Part model, mm, in its own coordinate system. A direction names the side the tool comes from. Coordinates: 2 decimals unless noted, no trailing zeros. Write each loop counter-clockwise with the first axis right and the second up, starting at its lowest first coordinate (ties: lowest second). Pieces come first, ordered by that corner, then holes. Notation, with made-up numbers: (2.5, 43.25) - (30.5, 43.25) arc R10 cw to (30.5, 50.25) - close; hole circle Ø2 at (-2, 5.25). An arc over 180 degrees is marked (long way). Write each question's results on one line, items separated by ' | '.
from build123d import *

# Parameters (mm, degrees)
SKETCH_W     = 108
SKETCH_H     = 75.2
PAD_DEPTH    = 2
SKETCH001_R  = 1.55
POCKET_DEPTH = 2
SKETCH002_W  = 10
SKETCH002_H  = 10
PAD001_DEPTH = 60
PAD002_DEPTH = 10
PAD003_DEPTH = 10
PAD004_DEPTH = 10
SKETCH003_W  = 10
SKETCH003_H  = 10
PAD005_DEPTH = 60
PAD006_DEPTH = 10
FILLET_R     = 1
FILLET001_R  = 1
FILLET002_R  = 1
FILLET003_R  = 1
BOX_W        = 108
BOX_H        = 75.2
BOX_DEPTH    = 10
BOX001_W     = 216
BOX001_H     = 150.4
BOX001_DEPTH = 30


with BuildPart() as part:
    # Sketch → Pad (new body)
    with BuildSketch(Plane.XY):
        Rectangle(SKETCH_W, SKETCH_H)
    extrude(amount=PAD_DEPTH)

    # Sketch001 (on Face6 of Pad) → Pocket (cut)
    with BuildSketch(Plane.XY.offset(2)):
        with Locations((-49.75, 33.05)):
            Circle(SKETCH001_R)
        with Locations((49.75, 33.05)):
            Circle(SKETCH001_R)
        with Locations((49.75, -33.05)):
            Circle(SKETCH001_R)
        with Locations((-49.75, -33.05)):
            Circle(SKETCH001_R)
    extrude(amount=-POCKET_DEPTH, mode=Mode.SUBTRACT)

    # Sketch002 (on Face5 of Pocket) → Pad001 (join)
    with BuildSketch(Plane(origin=(-14.437445, 5.037445, 35.081278), x_dir=(0.866025, 0, 0.5), z_dir=(-0.433013, 0.5, 0.75))):
        with Locations((-32.6, 32.6)):
            Rectangle(SKETCH002_W, SKETCH002_H)
    pad001 = extrude(amount=PAD001_DEPTH)

    # Mirrored: Pad001 across YZ
    add(pad001.mirror(Plane.YZ))

    # Mirrored001: Pad001 across XZ
    add(pad001.mirror(Plane.XZ))

    # Mirrored001 Face22 → Pad002 (add)
    with BuildSketch(Plane(origin=(34.284733, 32.964866, 5.00416), x_dir=(-0.755929, 0.654654, 0), z_dir=(-0.433013, -0.5, -0.75))):
        Polygon((3.146916, 4.541863), (-2.963185, 4.541863), (-7.030988, 1.019042), (-0.484451, -6.540247), (7.074838, 0.006289), align=None)
    extrude(amount=PAD002_DEPTH)

    # Pad002 Face21 → Pad003 (add)
    with BuildSketch(Plane(origin=(-34.284733, 32.964866, 5.00416), x_dir=(-0.755929, -0.654654, 0), z_dir=(0.433013, -0.5, -0.75))):
        Polygon((2.963185, 4.541863), (-3.146916, 4.541863), (-7.074838, 0.006289), (0.484451, -6.540247), (7.030988, 1.019042), align=None)
    extrude(amount=PAD003_DEPTH)

    # Pad003 Face35 → Pad004 (add)
    with BuildSketch(Plane(origin=(-34.284733, -32.964866, 5.00416), x_dir=(0.755929, -0.654654, 0), z_dir=(0.433013, 0.5, -0.75))):
        Polygon((3.146916, 4.541863), (-2.963185, 4.541863), (-7.030988, 1.019042), (-0.484451, -6.540247), (7.074838, 0.006289), align=None)
    extrude(amount=PAD004_DEPTH)

    # Sketch003 (on Face4 of Pad004) → Pad005 (join)
    with BuildSketch(Plane(origin=(14.437445, -5.037445, 35.081278), x_dir=(0.866025, 0, -0.5), z_dir=(0.433013, -0.5, 0.75))):
        with Locations((32.6, -32.6)):
            Rectangle(SKETCH003_W, SKETCH003_H)
    extrude(amount=PAD005_DEPTH)

    # Pad005 Face44 → Pad006 (add)
    with BuildSketch(Plane(origin=(34.284733, -32.964866, 5.00416), x_dir=(0.755929, 0.654654, 0), z_dir=(-0.433013, 0.5, -0.75))):
        Polygon((-7.074838, 0.006289), (0.484451, -6.540247), (7.030988, 1.019042), (2.963185, 4.541863), (-3.146916, 4.541863), align=None)
    extrude(amount=PAD006_DEPTH)

    # Fillet
    fillet_edges = [part.edges().sort_by_distance(p)[0] for p in [
        (-54, -37.6, 1),
    ]]
    fillet(fillet_edges, radius=FILLET_R)

    # Fillet001
    fillet001_edges = [part.edges().sort_by_distance(p)[0] for p in [
        (-54, 37.6, 1),
    ]]
    fillet(fillet001_edges, radius=FILLET001_R)

    # Fillet002
    fillet002_edges = [part.edges().sort_by_distance(p)[0] for p in [
        (54, -37.6, 1),
    ]]
    fillet(fillet002_edges, radius=FILLET002_R)

    # Fillet003
    fillet003_edges = [part.edges().sort_by_distance(p)[0] for p in [
        (54, 37.6, 1),
    ]]
    fillet(fillet003_edges, radius=FILLET003_R)

    # Box → Box (cut)
    with BuildSketch(Plane(origin=(-54, 37.6, 0), x_dir=(1, 0, 0), z_dir=(0, 0, -1))):
        with Locations((54, 37.6)):
            Rectangle(BOX_W, BOX_H)
    extrude(amount=BOX_DEPTH, mode=Mode.SUBTRACT)

    # Box001 → Box001 (cut)
    with BuildSketch(Plane(origin=(-108, -75.2, 32), x_dir=(1, 0, 0), z_dir=(0, 0, 1))):
        with Locations((108, 75.2)):
            Rectangle(BOX001_W, BOX001_H)
    extrude(amount=BOX001_DEPTH, mode=Mode.SUBTRACT)


solid = part.part
(1) Flat gauge pins, fed straight in: P1, Ø1, axis at y = -15, z = 1, coming from the +X side; P2, Ø3.5, axis at x = 49.75, y = 33.05, coming from the +Z side; P3, Ø1, axis at y = -45.5, z = 18.5, coming from the -X side. Where does each tip first touch, or does it go through?
Return value:
P1: stops at x = 54 | P2: stops at z = 2 | P3: stops at x = -48.57
(2) Saw through at B-B on x = -49.75. Write the cut outline in (y, z), then the cut area to 3 significant figures.
Return value:
outline: (-57.11, 32) - (-51.63, 21.04) - (-40.08, 21.04) - (-45.56, 32) - close; (-37.6, 0) - (-34.6, 0) - (-34.6, 2) - (-37.6, 2) - close; (-31.5, 0) - (31.5, 0) - (31.5, 2) - (-31.5, 2) - close; (34.6, 0) - (37.6, 0) - (37.6, 2) - (34.6, 2) - close; (40.08, 21.04) - (51.63, 21.04) - (57.11, 32) - (45.56, 32) - close | area: 391 mm^2
(3) 3-axis set-ups, long thin cutter, end or side, ignore diameter. For faces 1 (the flat face through (-28.834, 30.502, 4.817)), 2 (the flat face through (-43.706, -38.034, 20.436)), 3 (the flat face through (43.706, 38.034, 20.436)): which of +Z, -Z, +X, -X, +Y, -Y reach the whole face in a straight line?
Return value:
face 1: +Z, +Y, -Y | face 2: +Z, -X | face 3: +Z, +X
(4) Saw through at C-C on y = 18.5. Write the cut outline in (x, z), then the cut area to 3 significant figures.
Return value:
outline: (-54, 0) - (54, 0) - (54, 2) - (-54, 2) - close | area: 216 mm^2
(5) Wall check: line 1 (Y direction, x = -49.75, z = 1.5); line 2 (X direction, y = -33, z = 1); line 3 (Y direction, x = -49, z = 1). Give the ranges that are in metal, low to high. Write a range as from..to.
Return value:
line 1: y = -37.6..-34.6, -31.5..31.5, 34.6..37.6 | line 2: x = -54..-51.3, -48.2..48.2, 51.3..54 | line 3: y = -37.6..-34.41, -31.69..31.69, 34.41..37.6
(6) Two-plate mould, pull along Y, no slides. Class faces 4 (the flat face through (33.131, -27.074, 4.621)), 5 (the flat face through (42.439, 48.117, 18.241)), 6 (the flat face through (-50, -51, 32)): released by +Y, released by -Y, zero draft, split by the parting line, or undercut.
Return value:
face 4: undercut | face 5: released by +Y | face 6: zero draft
(7) Saw through at A-A on z = 27.5. Write the cut outline in (x, y), then the cut area to 3 significant figures.
Return value:
outline: (-53.48, -55.93) - (-41.93, -52.6) - (-41.93, -41.05) - (-53.48, -44.39) - close; (-53.48, 44.39) - (-41.93, 41.05) - (-41.93, 52.6) - (-53.48, 55.93) - close; (41.93, -52.6) - (53.48, -55.93) - (53.48, -44.39) - (41.93, -41.05) - close; (41.93, 41.05) - (53.48, 44.39) - (53.48, 55.93) - (41.93, 52.6) - close | area: 533 mm^2
(8) Saw through at D-D on x = 4.5. Write the cut outline in (y, z), then the cut area to 3 significant figures.
Return value:
outline: (-37.6, 0) - (37.6, 0) - (37.6, 2) - (-37.6, 2) - close | area: 150 mm^2
